Can you work these out from the model? Positions are in its coordinate system, mm. A direction names the side the tool comes from. Give positions to 0.01 mm unless a question says otherwise; leave off trailing zeros. Write each loop counter-clockwise with the first axis right and the second up, starting at its lowest first coordinate (ties: lowest second). Pieces come first, ordered by that corner, then holes. Notation, with made-up numbers: M 80.5,68 L 118.5,68 A14 cw 118.5,85 Z; hole C 63,87 d2. An arc over 180 degrees is marked long. Answer as CSV lines item,"result". Start each with the question number.
```python
from build123d import *

# Parameters (mm, degrees)
EXTRUDE_1_DEPTH      = 25
EXTRUDE_2_DEPTH      = 5
EXTRUDE_2_DEPTH_BACK = 20
SKETCH_2_R           = 0.775
FILLET_1_R           = 0.2
SKETCH_3_R           = 1.5
CUT_EXTRUDE_1_DEPTH  = 10


with BuildPart() as part:
    # 草图1 → 凸台-拉伸1 (new body)
    with BuildSketch(Plane(origin=(0, 0, 0), x_dir=(1, 0, 0), z_dir=(0, 1, 0))):
        with BuildLine():
            Line((-11.375, -7.85), (-10.875, -7.85))
            ThreePointArc((-10.875, -7.85), (-10.733578644, -7.791421356), (-10.675, -7.65))
            Line((-10.675, -7.65), (-10.675, -0.65))
            Line((-10.675, -0.65), (10.675, -0.65))
            Line((10.675, -0.65), (10.675, -7.65))
            ThreePointArc((10.675, -7.65), (10.733578644, -7.791421356), (10.875, -7.85))
            Line((10.875, -7.85), (11.375, -7.85))
            ThreePointArc((11.375, -7.85), (11.516421356, -7.791421356), (11.575, -7.65))
            Line((11.575, -7.65), (11.575, 7.65))
            ThreePointArc((11.575, 7.65), (11.516421356, 7.791421356), (11.375, 7.85))
            Line((11.375, 7.85), (10.875, 7.85))
            ThreePointArc((10.875, 7.85), (10.733578644, 7.791421356), (10.675, 7.65))
            Line((10.675, 7.65), (10.675, 3.55))
            ThreePointArc((10.675, 3.55), (10.616421356, 3.408578644), (10.475, 3.35))
            Line((10.475, 3.35), (9.558099354, 3.35))
            ThreePointArc((9.558099354, 3.35), (9.416677998, 3.291421356), (9.358099354, 3.15))
            Line((9.358099354, 3.15), (9.358099354, 2.212306229))
            ThreePointArc((9.358099354, 2.212306229), (9.190112859, 0.773679762), (8.358099354, 1.959267845))
            Line((8.358099354, 1.959267845), (8.358099354, 3.15))
            ThreePointArc((8.358099354, 3.15), (8.29952071, 3.291421356), (8.158099354, 3.35))
            Line((8.158099354, 3.35), (7.325, 3.35))
            ThreePointArc((7.325, 3.35), (7.183578644, 3.408578644), (7.125, 3.55))
            Line((7.125, 3.55), (7.125, 7.65))
            ThreePointArc((7.125, 7.65), (7.066421356, 7.791421356), (6.925, 7.85))
            Line((6.925, 7.85), (6.425, 7.85))
            ThreePointArc((6.425, 7.85), (6.283578644, 7.791421356), (6.225, 7.65))
            Line((6.225, 7.65), (6.225, 3.55))
            ThreePointArc((6.225, 3.55), (6.166421356, 3.408578644), (6.025, 3.35))
            Line((6.025, 3.35), (2.875, 3.35))
            ThreePointArc((2.875, 3.35), (2.733578644, 3.408578644), (2.675, 3.55))
            Line((2.675, 3.55), (2.675, 7.65))
            ThreePointArc((2.675, 7.65), (2.616421356, 7.791421356), (2.475, 7.85))
            Line((2.475, 7.85), (1.975, 7.85))
            ThreePointArc((1.975, 7.85), (1.833578644, 7.791421356), (1.775, 7.65))
            Line((1.775, 7.65), (1.775, 3.55))
            ThreePointArc((1.775, 3.55), (1.716421356, 3.408578644), (1.575, 3.35))
            Line((1.575, 3.35), (0.7, 3.35))
            ThreePointArc((0.7, 3.35), (0.558578644, 3.291421356), (0.5, 3.15))
            Line((0.5, 3.15), (0.5, 2.829795897))
            ThreePointArc((0.5, 2.829795897), (0, 0.75), (-0.5, 2.829795897))
            Line((-0.5, 2.829795897), (-0.5, 3.15))
            ThreePointArc((-0.5, 3.15), (-0.558578644, 3.291421356), (-0.7, 3.35))
            Line((-0.7, 3.35), (-1.575, 3.35))
            ThreePointArc((-1.575, 3.35), (-1.716421356, 3.408578644), (-1.775, 3.55))
            Line((-1.775, 3.55), (-1.775, 7.65))
            ThreePointArc((-1.775, 7.65), (-1.833578644, 7.791421356), (-1.975, 7.85))
            Line((-1.975, 7.85), (-2.475, 7.85))
            ThreePointArc((-2.475, 7.85), (-2.616421356, 7.791421356), (-2.675, 7.65))
            Line((-2.675, 7.65), (-2.675, 3.55))
            ThreePointArc((-2.675, 3.55), (-2.733578644, 3.408578644), (-2.875, 3.35))
            Line((-2.875, 3.35), (-6.025, 3.35))
            ThreePointArc((-6.025, 3.35), (-6.166421356, 3.408578644), (-6.225, 3.55))
            Line((-6.225, 3.55), (-6.225, 7.65))
            ThreePointArc((-6.225, 7.65), (-6.283578644, 7.791421356), (-6.425, 7.85))
            Line((-6.425, 7.85), (-6.925, 7.85))
            ThreePointArc((-6.925, 7.85), (-7.066421356, 7.791421356), (-7.125, 7.65))
            Line((-7.125, 7.65), (-7.125, 3.55))
            ThreePointArc((-7.125, 3.55), (-7.183578644, 3.408578644), (-7.325, 3.35))
            Line((-7.325, 3.35), (-8.37016684, 3.35))
            ThreePointArc((-8.37016684, 3.35), (-8.511588196, 3.291421356), (-8.57016684, 3.15))
            Line((-8.57016684, 3.15), (-8.57016684, 2.169878635))
            ThreePointArc((-8.57016684, 2.169878635), (-8.907689329, 0.755517226), (-9.57016684, 2.049914064))
            Line((-9.57016684, 2.049914064), (-9.57016684, 3.15))
            ThreePointArc((-9.57016684, 3.15), (-9.628745484, 3.291421356), (-9.77016684, 3.35))
            Line((-9.77016684, 3.35), (-10.475, 3.35))
            ThreePointArc((-10.475, 3.35), (-10.616421356, 3.408578644), (-10.675, 3.55))
            Line((-10.675, 3.55), (-10.675, 7.65))
            ThreePointArc((-10.675, 7.65), (-10.733578644, 7.791421356), (-10.875, 7.85))
            Line((-10.875, 7.85), (-11.375, 7.85))
            ThreePointArc((-11.375, 7.85), (-11.516421356, 7.791421356), (-11.575, 7.65))
            Line((-11.575, 7.65), (-11.575, -7.65))
            ThreePointArc((-11.575, -7.65), (-11.516421356, -7.791421356), (-11.375, -7.85))
        make_face()
    extrude(amount=EXTRUDE_1_DEPTH)

    # 草图2 → 凸台-拉伸2 (add, two sides: drawn at the far end of the back side and taken through both)
    with BuildSketch(Plane.XZ.offset(-EXTRUDE_2_DEPTH_BACK)):
        with Locations(Location((-9, -1.525, 0), (0, 0, 270))):
            Circle(SKETCH_2_R)
        with Locations(Location((9, -1.525, 0), (0, 0, 270))):
            Circle(SKETCH_2_R)
    extrude(amount=EXTRUDE_2_DEPTH + EXTRUDE_2_DEPTH_BACK)

    # 圆角1
    fillet_1_edges = [part.edges().sort_by_distance(p)[0] for p in [
        (-10.675, 12.5, 0.65),
        (10.675, 12.5, 0.65),
    ]]
    fillet(fillet_1_edges, radius=FILLET_1_R)

    # 草图3 → 切除-拉伸1 (cut)
    with BuildSketch(Plane.XY.offset(0.65)):
        with Locations((0, 18.5)):
            Circle(SKETCH_3_R)
    extrude(amount=-CUT_EXTRUDE_1_DEPTH, mode=Mode.SUBTRACT)


solid = part.part
```
1) I'm going to push flat-ended pins straight in: P1, Ø6, axis at x = -4.5, z = 1, coming from the -Y side; P2, Ø10, axis at x = -6, y = 20, coming from the +Z side; P3, Ø0.6, axis at x = -10.5, y = 10, coming from the -Z side; P4, Ø6, axis at x = -3, y = 9.5, coming from the +Z side. Where does each tip first touch, or does it pass through?
2) Thinking about a two-plate mould opening in X: for faces 1 (the cylindrical face through (0.04, 22.22, -0.75)), 2 (the flat face through (-9, -5, -2)), which applies, released by +X, released by -X, zero draft, split by the parting line, or undercut?
3) I need wall thicknesses on L1, parallel to X at y = 11.5, z = -3.5 (3 decimals); L2, parallel to X at y = 5, z = 5 (3 decimals); L3, parallel to X at y = 22, z = -1.85 (3 decimals). Which ranges of each line are inside material? Lowest first, please. Write a range as from..to.
4) I want a section at D-D, the plane z = 0. Please give me the cut outline in (x, y) (3 decimals).
5) I want a section at A-A, the plane z = -4. Please give me the cut outline in (x, y) (3 decimals).
6) I want a section at B-B, the plane x = 0. Please give me the cut outline in (y, z).
7) On a 3-axis mill with a long thin cutter (end or side, diameter ignored), from which of +Z, -Z, +X, -X, +Y, -Y can I reach the whole of each face in a straight line? I mean faces 3 (the flat face through (0, 12, 0.65)), 4 (the flat face through (-8, 12, -3.35)), 5 (the flat face through (9, 20, -2)). Say none if no direction works.
8) I want a section at C-C, the plane y = -2. Please give me the cut outline in (x, z) (3 decimals), then the cut area to 3 significant figures.
Values found:
1,P1,"stops at y = 0"
1,P2,"stops at z = 7.85"
1,P3,"stops at z = -7.84"
1,P4,"stops at z = 0.65"
2,face 1,"undercut"
2,face 2,"zero draft"
3,L1,"x = -11.575..-10.669, -7.131..-6.219, -2.681..-1.769, 1.769..2.681, 6.219..7.131, 10.669..11.575"
3,L2,"x = -11.575..-10.675, 10.675..11.575"
3,L3,"x = -11.575..-9.704, -8.296..-1.1, 1.1..8.296, 9.704..11.575"
4,outline,"M -11.575,0 L 11.575,0 L 11.575,25 L -11.575,25 Z; hole C 0,18.5 d3"
5,outline,"M -11.575,0 L -10.675,0 L -10.675,25 L -11.575,25 Z; M -7.125,0 L -6.225,0 L -6.225,25 L -7.125,25 Z; M -2.675,0 L -1.775,0 L -1.775,25 L -2.675,25 Z; M 1.775,0 L 2.675,0 L 2.675,25 L 1.775,25 Z; M 6.225,0 L 7.125,0 L 7.125,25 L 6.225,25 Z; M 10.675,0 L 11.575,0 L 11.575,25 L 10.675,25 Z"
6,outline,"M 0,-0.75 L 17,-0.75 L 17,0.65 L 0,0.65 Z; M 20,-0.75 L 25,-0.75 L 25,0.65 L 20,0.65 Z"
7,face 3,"+Z, +Y, -Y"
7,face 4,"-Z, +Y, -Y"
7,face 5,"+Y"
8,outline,"C -9,-1.525 d1.55; C 9,-1.525 d1.55"
8,area,"3.77 mm²"
